Input: part model. Units: mm. Frame: model coordinates. Coordinates: 2 decimals unless noted, no trailing zeros. Loops run counter-clockwise (first coordinate to the right, second up) from the corner with the lowest first, then second, coordinate; pieces in that order, holes last. Notation, with made-up numbers: (65.5, -26) - (122.5, -26) arc R16 ccw to (122.5, -18) - close; hole circle Ø11 at (75.5, 26.25). An arc over 180 degrees is marked (long way). Use a Markdown table: item, result. Add a question column.
1. Section query C-C on x = 38.1. Return the cut outline in (y, z) (3 decimals), then the cut area to 3 significant figures.
2. Section query A-A on y = 2.1. Return the cut outline in (x, z) (3 decimals).
3. Section query D-D on z = -14. Return the cut outline in (x, y) (3 decimals), then the cut area to 3 significant figures.
4. Contact query for flat-ended pins moving along their axis: P1, Ø23, axis at x = 38.1, z = -120.65, coming from the +Y side (3 decimals); P2, Ø1, axis at y = 2, z = -33, coming from the -X side (3 decimals); P3, Ø1, axis at y = 2.5, z = -115, coming from the +X side (3 decimals). Output: stop coordinate, or through.
5. Ray query, L1, parallel to X at y = 1.6, z = -120.65 (3 decimals); L2, parallel to X at y = 0.55, z = -100.5 (3 decimals); L3, parallel to X at y = 1.5, z = -125.5 (3 decimals). Return the intervals inside material, ascending. Write a range as [from, to].
6. Section query B-B on z = -120.65. Return the cut outline in (x, y) (3 decimals), then the cut area to 3 significant figures.
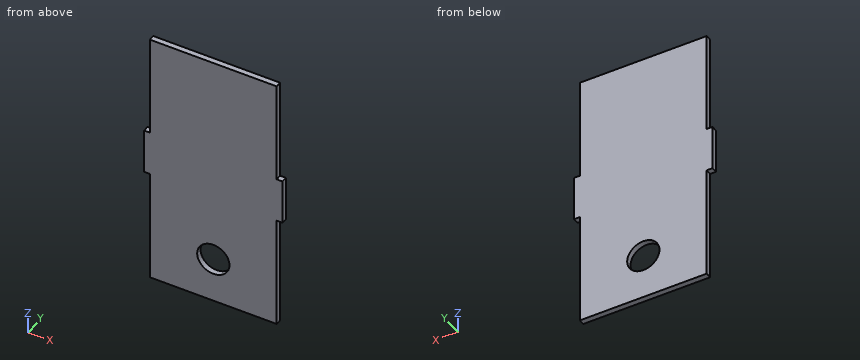
```python
from build123d import *

# Parameters (mm, degrees)
SKETCH1_W           = 76.2
SKETCH1_H           = 146.05
SKETCH1_R           = 8.89
BOSS_EXTRUDE1_DEPTH = 3.175
SKETCH2_W           = 3.175
SKETCH2_H           = 57.15
SKETCH2_H_2         = 63.5
CUT_EXTRUDE1_DEPTH  = 3.175


with BuildPart() as part:
    # Sketch1 → Boss-Extrude1 (new body)
    with BuildSketch(Plane(origin=(0, 0, 0), x_dir=(1, 0, 0), z_dir=(0, 1, 0))):
        with Locations((38.1, 73.025)):
            Rectangle(SKETCH1_W, SKETCH1_H)
        with Locations(Location((38.1, 120.65, 0), (0, 0, 270))):
            Circle(SKETCH1_R, mode=Mode.SUBTRACT)
    extrude(amount=BOSS_EXTRUDE1_DEPTH)

    # Sketch2 → Cut-Extrude1 (cut)
    with BuildSketch(Plane(origin=(0, 3.175, 0), x_dir=(1, 0, 0), z_dir=(0, 1, 0))):
        with Locations((1.5875, 28.575)):
            Rectangle(SKETCH2_W, SKETCH2_H)
        with Locations((1.5875, 114.3)):
            Rectangle(SKETCH2_W, SKETCH2_H_2)
        with Locations((74.6125, 114.3)):
            Rectangle(SKETCH2_W, SKETCH2_H_2)
        with Locations((74.6125, 28.575)):
            Rectangle(SKETCH2_W, SKETCH2_H)
    extrude(amount=-CUT_EXTRUDE1_DEPTH, mode=Mode.SUBTRACT)


solid = part.part
```
Resolved:
| question | item | result |
|---|---|---|
| 1 | outline | (0, -146.05) - (3.175, -146.05) - (3.175, -129.54) - (0, -129.54) - close; (0, -111.76) - (3.175, -111.76) - (3.175, 0) - (0, 0) - close |
| 1 | area | 407 mm² |
| 2 | outline | (0, -82.55) - (3.175, -82.55) - (3.175, -146.05) - (73.025, -146.05) - (73.025, -82.55) - (76.2, -82.55) - (76.2, -57.15) - (73.025, -57.15) - (73.025, 0) - (3.175, 0) - (3.175, -57.15) - (0, -57.15) - close; hole circle Ø17.78 at (38.1, -120.65) |
| 3 | outline | (3.175, 0) - (73.025, 0) - (73.025, 3.175) - (3.175, 3.175) - close |
| 3 | area | 222 mm² |
| 4 | P1 | y = 3.175 |
| 4 | P2 | x = 3.175 |
| 4 | P3 | x = 73.025 |
| 5 | L1 | [3.175, 29.21], [46.99, 73.025] |
| 5 | L2 | [3.175, 73.025] |
| 5 | L3 | [3.175, 30.65], [45.55, 73.025] |
| 6 | outline | (3.175, 0) - (29.21, 0) - (29.21, 3.175) - (3.175, 3.175) - close; (46.99, 0) - (73.025, 0) - (73.025, 3.175) - (46.99, 3.175) - close |
| 6 | area | 165 mm² |
